Source: three-view drawing plus pictorial views. Frame: mm from the lowest corner of the part. Give positions to 0.01 mm unless a question says otherwise; leave off trailing zeros. Loops run counter-clockwise (first coordinate to the right, second up) from the corner with the lowest first, then second, coordinate; pieces in that order, holes last. Notation, with made-up numbers: (-40, 52) - (7, 52) arc R16 cw to (7, 68) - close; hole circle Ø4 at (-17.5, 46). An arc over 180 degrees is marked (long way). Answer in a Markdown table with one row per item.
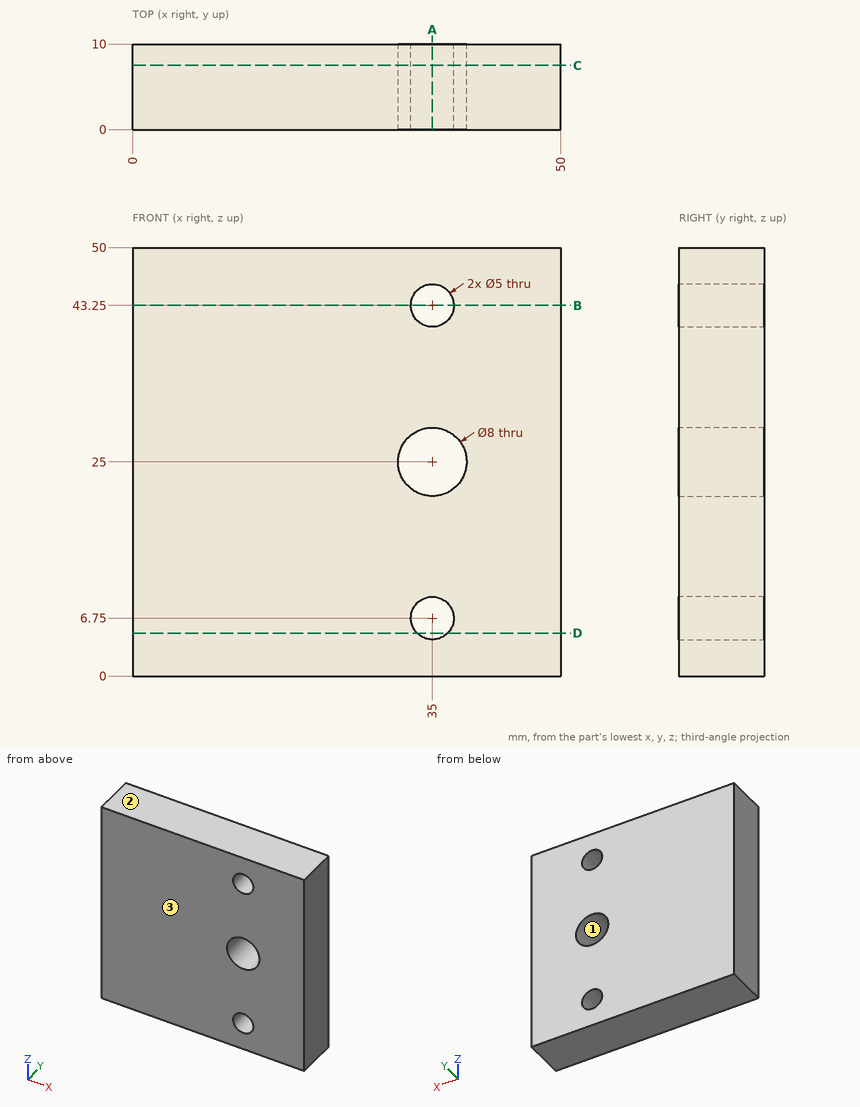
Q1. First-contact query: pin 1 (3 mm diameter, centred on x = 35, z = 43.25, fed in from +Y). Flat tip, straight axial feed; report the tip coordinate or a pass-through.
Check values:
| item | result |
|---|---|
| pin 1 | through |
Q2. Cut plane B-B (z = 43.25). Output: boundary loops of the cut face in (x, y).
Check values:
| item | result |
|---|---|
| outline | (0, 0) - (32.5, 0) - (32.5, 10) - (0, 10) - close; (37.5, 0) - (50, 0) - (50, 10) - (37.5, 10) - close |
Q3. Cut plane D-D (z = 5). Output: boundary loops of the cut face in (x, y).
Check values:
| item | result |
|---|---|
| outline | (0, 0) - (33.21, 0) - (33.21, 10) - (0, 10) - close; (36.79, 0) - (50, 0) - (50, 10) - (36.79, 10) - close |
Q4. Material intervals for line 1 along X through (y, z) = (4.25, 25); line 2 along X through (y, z) = (2.75, 43.25); line 3 along Z through (x, y) = (36, 5.25), sorted ascending.
Check values:
| item | result |
|---|---|
| line 1 | 0 to 31, 39 to 50 |
| line 2 | 0 to 32.5, 37.5 to 50 |
| line 3 | 0 to 4.46, 9.04 to 21.13, 28.87 to 40.96, 45.54 to 50 |
Q5. Draft query along Z for the marked faces 1, 2 and 3. Return one class per face: pulls with the +Z half, pulls with the -Z half, needs draft (parallel to the pull), parting line crosses it, or undercut.
Check values:
| item | result |
|---|---|
| face 1 | undercut |
| face 2 | pulls with the +Z half |
| face 3 | needs draft |
Q6. Cut plane A-A (x = 35). Output: boundary loops of the cut face in (y, z).
Check values:
| item | result |
|---|---|
| outline | (0, 0) - (10, 0) - (10, 4.25) - (0, 4.25) - close; (0, 9.25) - (10, 9.25) - (10, 21) - (0, 21) - close; (0, 29) - (10, 29) - (10, 40.75) - (0, 40.75) - close; (0, 45.75) - (10, 45.75) - (10, 50) - (0, 50) - close |
Q7. Cut plane C-C (y = 7.5). Output: boundary loops of the cut face in (x, z), and give its area (3 significant figures).
Check values:
| item | result |
|---|---|
| outline | (0, 0) - (50, 0) - (50, 50) - (0, 50) - close; hole circle Ø8 at (35, 25); hole circle Ø5 at (35, 6.75); hole circle Ø5 at (35, 43.25) |
| area | 2,410 mm² |
